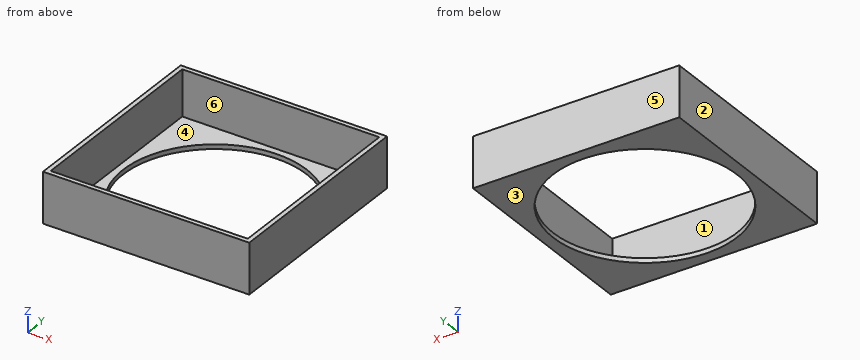
```python
from build123d import *

# Parameters (mm, degrees)
F0_W      = 114.3
F0_H      = 114.3
F1_DEPTH  = 2.54
F2_W      = 114.3
F2_H      = 25.4
F3_DEPTH  = 2.54
F5_W      = 109.22
F5_H      = 25.4
F6_DEPTH  = 2.54
F8_W      = 114.3
F8_H      = 114.3
F8_W_2    = 109.22
F8_H_2    = 109.22
F9_DEPTH  = 2.54
F10_W     = 114.3
F10_H     = 114.3
F11_DEPTH = 2.54
F12_W     = 76.2
F12_H     = 104.14
F13_DEPTH = 1.27
F14_R     = 6.35
F15_DEPTH = 1.27
F17_R     = 50.8982940966
F18_DEPTH = 2.54


with BuildPart() as f1:
    # F0 (on Top) → F1 (new body)
    with BuildSketch(Plane.XY):
        Rectangle(F0_W, F0_H)
    extrude(amount=F1_DEPTH)

    # F4: F3 across plane


with BuildPart() as f3:
    # F2 (on face) → F3 (new body)
    with BuildSketch(Plane.YZ.offset(57.15)):
        with Locations((0, 15.24)):
            Rectangle(F2_W, F2_H)
    extrude(amount=-F3_DEPTH)


with BuildPart() as f1_1:
    add(f1.part)
    add(f3.part.mirror(Plane.YZ))



with BuildPart() as f6:
    # F5 (on face) → F6 (new body)
    with BuildSketch(Plane(origin=(0, 57.15, 0), x_dir=(-1, 0, 0), z_dir=(0, 1, 0))):
        with Locations((0, 15.24)):
            Rectangle(F5_W, F5_H)
    extrude(amount=-F6_DEPTH)


with BuildPart() as f1_2:
    add(f1_1.part)

    add(f3.part)  # F7 merges F3

    add(f6.part)  # F7 merges F6
    # F7: F6 across plane
    add(f6.part.mirror(Plane.XZ))

    # F17 (on face) → F18 (cut, through all)
    with BuildSketch(Plane.XY.offset(2.54)):
        Circle(F17_R)
    extrude(amount=-F18_DEPTH, mode=Mode.SUBTRACT)


with BuildPart() as f9:
    # F8 (on face) → F9 (new body)
    with BuildSketch(Plane.XY.offset(27.94)):
        Rectangle(F8_W, F8_H)
        Rectangle(F8_W_2, F8_H_2, mode=Mode.SUBTRACT)
        Rectangle(F8_W_2, F8_H_2)
    extrude(amount=F9_DEPTH)

    # F10 (on face) → F11 (join)
    with BuildSketch(Plane.XY.offset(30.48)):
        Rectangle(F10_W, F10_H)
    extrude(amount=F11_DEPTH)

    # F12 (on face) → F13 (cut)
    with BuildSketch(Plane.XY.offset(33.02)):
        with Locations((-13.97, 0)):
            Rectangle(F12_W, F12_H)
    extrude(amount=-F13_DEPTH, mode=Mode.SUBTRACT)

    # F14 (on face) → F15 (cut)
    with BuildSketch(Plane.XY.offset(33.02)):
        with BuildLine():
            ThreePointArc((55.245, 45.72), (48.895, 52.07), (42.545, 45.72))
            ThreePointArc((42.545, 45.72), (48.895, 39.37), (55.245, 45.72))
        make_face()
        with Locations((32.385, 45.72)):
            Circle(F14_R)
        with BuildLine():
            ThreePointArc((40.64, 6.35), (36.1498719395, -4.4901280605), (46.99, 0))
            ThreePointArc((46.99, 0), (45.1301280605, 4.4901280605), (40.64, 6.35))
        make_face()
    extrude(amount=-F15_DEPTH, mode=Mode.SUBTRACT)


solid = f1_2.part
```
Could you check a few things on this model? Use its own coordinates, in mm. Face numbers are marked on the shaded views. A direction names the side the tool comes from. Coordinates: 2 decimals unless noted, no trailing zeros. Order: outer loops, then holes, each group sorted by start corner. A loop starts at its lowest first (then second) coordinate and runs counter-clockwise, first axis right, second up. Notation, with made-up numbers: M -20.75,-29.75 L 27.25,-29.75 A28 ccw 27.25,9.25 Z; hole C 53,72.25 d10. An arc over 180 degrees is marked long. Use one line per item in the form item = value. Start each with the question number.
1. Suppose I cut it at C-C on z = 6. Write out the boundary of the cut face in (x, y), then the cut area to 3 significant figures.
2. Please list where these lines run through material, in increasing order: line 1 (Y direction, x = -7.5, z = 22); line 2 (Y direction, x = 0, z = 1.3).
3. On a 3-axis mill with a long thin cutter (end or side, diameter ignored), from which of +Z, -Z, +X, -X, +Y, -Y can I reach the whole of each face in a straight line? I mean the marked faces 1 and 2. Say none if no direction works.
4. Suppose I cut it at A-A on x = 0. Write out the boundary of the cut face in (y, z), then the cut area to 3 significant figures.
5. We'd pull the mould along Y, two halves only. Please class the marked faces 3, 4, 5 and 6: +Y half, -Y half, draft (parallel to the pull), parting line (faces both ways), or undercut.
Geometry says:
q1.outline = M -57.15,-57.15 L 57.15,-57.15 L 57.15,57.15 L -57.15,57.15 Z; hole M -54.61,-54.61 L 54.61,-54.61 L 54.61,54.61 L -54.61,54.61 Z
q1.area = 1,140 mm^2
q2.line_1 = -57.15 to -54.61, 54.61 to 57.15
q2.line_2 = -57.15 to -50.9, 50.9 to 57.15
q3.face_1 = +Z
q3.face_2 = +Z, -Z, -X, +Y, -Y
q4.outline = M -57.15,0 L -50.9,0 L -50.9,2.54 L -54.61,2.54 L -54.61,27.94 L -57.15,27.94 Z; M 50.9,0 L 57.15,0 L 57.15,27.94 L 54.61,27.94 L 54.61,2.54 L 50.9,2.54 Z
q4.area = 161 mm^2
q5.face_3 = draft
q5.face_4 = undercut
q5.face_5 = +Y half
q5.face_6 = undercut
